Part print with two shaded views. Sizes in mm from the minimum x, y, z corner. Round coordinates to 2 decimals unless told otherwise and drop trailing zeros. Loops run counter-clockwise (first coordinate to the right, second up) from the corner with the lowest first, then second, coordinate; pieces in that order, holes last. Notation, with made-up numbers: (34, -7) -> (82, -7) arc R29 ccw to (82, 13) -> close; hole circle Ø6 at (-34, -39). An arc over 180 degrees is marked (long way). Use a Markdown table: item, result. Add a question column.
Item 1: Flat gauge pin, fed straight in: pin 1 (2.5 mm diameter, centred on x = 6.5, z = 63.5, fed in from -Y). Where does the tip first touch, or does it go through?
Item 2: Probe line 1 (Z direction, x = 53.5, y = 1.25); line 2 (X direction, y = 0.5, z = 63.5); line 3 (X direction, y = 0.6, z = 7). List the from-to ranges inside material, lowest first. Write a range as [from, to].
Item 3: Cut at A-A, the plane x = 6.5. List the corners of the cut face in (y, z).
Item 4: Cut at B-B, the plane z = 6.5. List the corners of the cut face in (x, y).
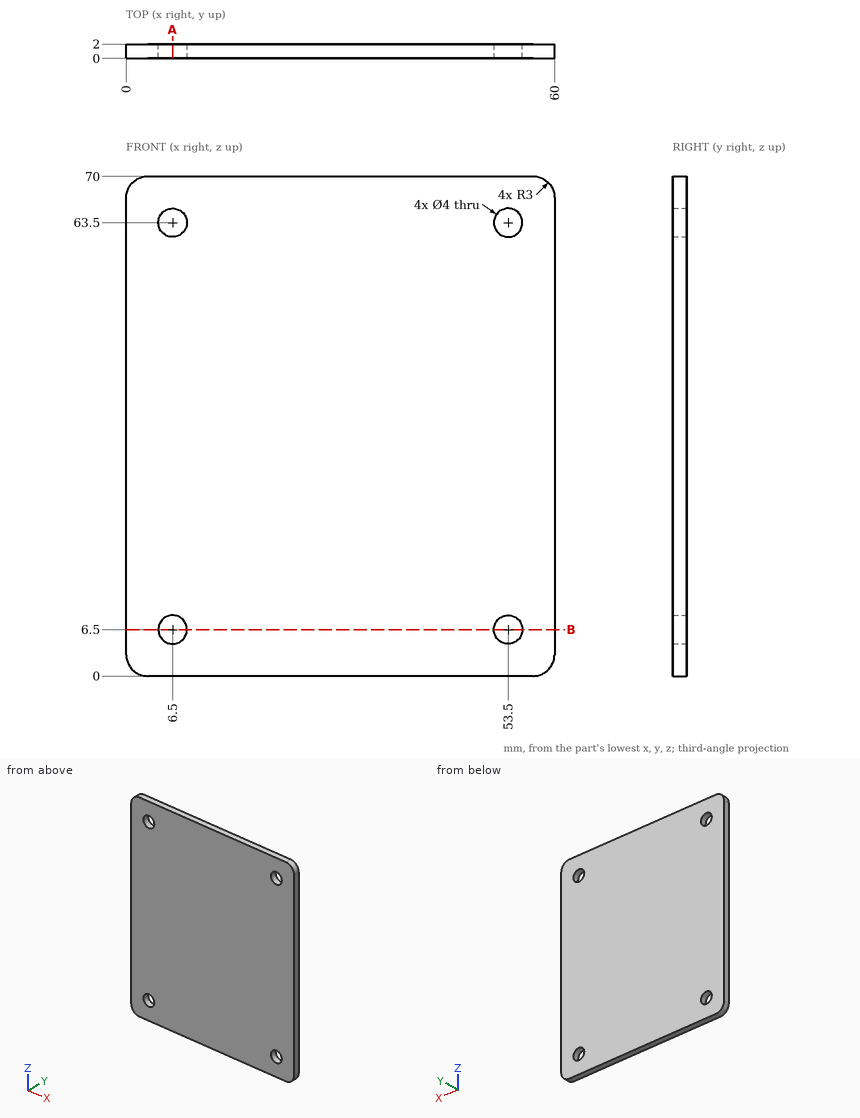
A:
| question | item | result |
|---|---|---|
| 1 | pin 1 | passes through |
| 2 | line 1 | z = [0, 4.5], [8.5, 61.5], [65.5, 70] |
| 2 | line 2 | x = [0, 4.5], [8.5, 51.5], [55.5, 60] |
| 2 | line 3 | x = [0, 4.56], [8.44, 51.56], [55.44, 60] |
| 3 | outline | (0, 0) -> (2, 0) -> (2, 4.5) -> (0, 4.5) -> close; (0, 8.5) -> (2, 8.5) -> (2, 61.5) -> (0, 61.5) -> close; (0, 65.5) -> (2, 65.5) -> (2, 70) -> (0, 70) -> close |
| 4 | outline | (0, 0) -> (4.5, 0) -> (4.5, 2) -> (0, 2) -> close; (8.5, 0) -> (51.5, 0) -> (51.5, 2) -> (8.5, 2) -> close; (55.5, 0) -> (60, 0) -> (60, 2) -> (55.5, 2) -> close |
